Source: CAD feature listing. Evaluate the final solid. Frame: model axes, mm. Face numbers are marked on the shaded views. A direction names the side the tool comes from. Coordinates: 2 decimals unless noted, no trailing zeros. Order: outer loops, then holes, each group sorted by start corner. A loop starts at its lowest first (then second) coordinate and runs counter-clockwise, first axis right, second up.
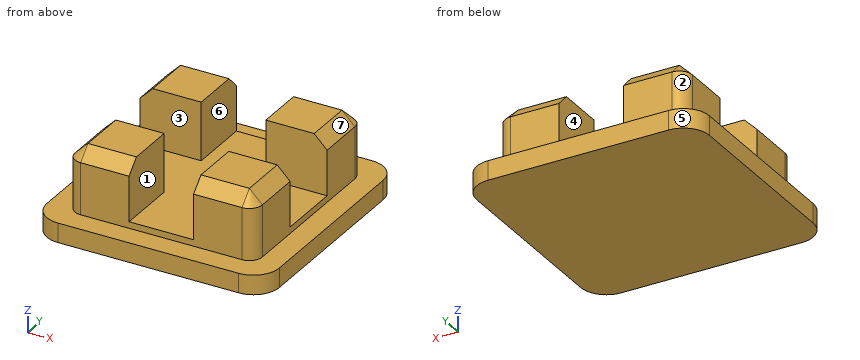
```python
from build123d import *

# Parameters (mm, degrees)
F1_DEPTH = 3
F3_DEPTH = 10
F5_DEPTH = 9
F6_SIZE  = 1.99999


# Not quite as in the source:
# - a fillet or chamfer is up to 0.001 mm smaller than in the source, because OpenCascade refuses the exact size


with BuildPart() as f1:
    # F0 (on Top) → F1 (new body)
    with BuildSketch(Plane.XY):
        with BuildLine():
            Line((16.3916659281, 18.4843443355), (-11.6083340719, 18.4843443355))
            ThreePointArc((-11.6083340719, 18.4843443355), (-14.4367611967, 17.3127714603), (-15.6083340719, 14.4843443355))
            Line((-15.6083340719, 14.4843443355), (-15.6083340719, -13.5156556645))
            ThreePointArc((-15.6083340719, -13.5156556645), (-14.4367611967, -16.3440827892), (-11.6083340719, -17.5156556645))
            Line((-11.6083340719, -17.5156556645), (16.3916659281, -17.5156556645))
            ThreePointArc((16.3916659281, -17.5156556645), (19.2200930528, -16.3440827892), (20.3916659281, -13.5156556645))
            Line((20.3916659281, -13.5156556645), (20.3916659281, 14.4843443355))
            ThreePointArc((20.3916659281, 14.4843443355), (19.2200930528, 17.3127714603), (16.3916659281, 18.4843443355))
        make_face()
    extrude(amount=F1_DEPTH)

    # F2 (on face) → F3 (join)
    with BuildSketch(Plane.XY.offset(3)):
        with BuildLine():
            Line((14.8916659281, 14.9843443355), (-10.1083340719, 14.9843443355))
            ThreePointArc((-10.1083340719, 14.9843443355), (-11.5225476343, 14.3985578979), (-12.1083340719, 12.9843443355))
            Line((-12.1083340719, 12.9843443355), (-12.1083340719, -12.0156556645))
            ThreePointArc((-12.1083340719, -12.0156556645), (-11.5225476343, -13.4298692268), (-10.1083340719, -14.0156556645))
            Line((-10.1083340719, -14.0156556645), (14.8916659281, -14.0156556645))
            ThreePointArc((14.8916659281, -14.0156556645), (16.3058794904, -13.4298692268), (16.8916659281, -12.0156556645))
            Line((16.8916659281, -12.0156556645), (16.8916659281, 12.9843443355))
            ThreePointArc((16.8916659281, 12.9843443355), (16.3058794904, 14.3985578979), (14.8916659281, 14.9843443355))
        make_face()
    extrude(amount=F3_DEPTH)

    # F4 (on face) → F5 (cut)
    with BuildSketch(Plane.XY.offset(13)):
        Polygon((7.3916660622, 14.9843443355), (-2.6083340719, 14.9843443355), (-2.6083340719, 5.4843444377), (-12.1083340719, 5.4843444377), (-12.1083340719, -4.5156556645), (-2.6083340719, -4.5156556645), (-2.6083340719, -14.0156556645), (7.3916660622, -14.0156556645), (7.3916660622, -4.5156556645), (16.8916659281, -4.5156556645), (16.8916659281, 5.4843444377), (7.3916660622, 5.4843444377), align=None)
    extrude(amount=-F5_DEPTH, mode=Mode.SUBTRACT)

    # F6 (size 2 in the source; OpenCascade refuses exactly that, so slightly less here)
    f6_edges = [f1.edges().sort_by_distance(p)[0] for p in [
        (11.141666, -14.015656, 13),
        (-6.358334, -14.015656, 13),
        (16.891666, 9.234344, 13),
        (-12.108334, 9.234344, 13),
    ]]
    chamfer(f6_edges, length=F6_SIZE)


solid = f1.part
```
1. Section query C-C, the plane y = -8.5. Output: boundary loops of the cut face in (x, z).
2. Contact query for flat-ended pins moving along their axis: P1, Ø6.5, axis at x = 8, z = 8, coming from the +Y side; P2, Ø4.5, axis at y = -11.5, z = 9, coming from the +X side; P3, Ø2.5, axis at y = -9, z = 10.5, coming from the -X side. Output: stop coordinate, or through.
3. Section query B-B, the plane x = 8. Output: boundary loops of the cut face in (y, z), plus the area to 3 significant figures.
4. Section query A-A, the plane z = 5.25. Output: boundary loops of the cut face in (x, y), plus the area to 3 significant figures.
5. Material intervals for line 1 along Y through (x, z) = (-6.5, 10.5); line 2 along X through (y, z) = (8, 4.5); line 3 along X through (y, z) = (-7, 11.5), sorted ascending.
6. Access query for the marked faces 1, 2 and 3. Directions: +Z, -Z, +X, -X, +Y, -Y. A direction counts if a zero-diameter tool reaches every point of the face in a straight line with its end or side. Return the directions, or none.
7. Section query D-D, the plane x = 2. Output: boundary loops of the cut face in (y, z), plus the area to 3 significant figures.
8. Draft query along X for the marked faces 4, 5, 6 and 7. Return one class per face: +X half, -X half, draft (parallel to the pull), parting line (faces both ways), or undercut.
Answer key:
1. outline: (-15.61, 0) - (20.39, 0) - (20.39, 3) - (16.89, 3) - (16.89, 11) - (14.89, 13) - (7.39, 13) - (7.39, 4) - (-2.61, 4) - (-2.61, 13) - (-10.11, 13) - (-12.11, 11) - (-12.11, 3) - (-15.61, 3) - close
2. P1: stops at y = 14.98
2. P2: stops at x = 16.89
2. P3: stops at x = -12.11
3. outline: (-17.52, 0) - (18.48, 0) - (18.48, 3) - (14.98, 3) - (14.98, 11) - (12.98, 13) - (5.48, 13) - (5.48, 4) - (-4.52, 4) - (-4.52, 13) - (-12.02, 13) - (-14.02, 11) - (-14.02, 3) - (-17.52, 3) - close
3. area: 304 mm2
4. outline: (-12.11, -12.02) arc R2 ccw to (-10.11, -14.02) - (-2.61, -14.02) - (-2.61, -4.52) - (-12.11, -4.52) - close; (-12.11, 5.48) - (-2.61, 5.48) - (-2.61, 14.98) - (-10.11, 14.98) arc R2 ccw to (-12.11, 12.98) - close; (7.39, -14.02) - (14.89, -14.02) arc R2 ccw to (16.89, -12.02) - (16.89, -4.52) - (7.39, -4.52) - close; (7.39, 5.48) - (16.89, 5.48) - (16.89, 12.98) arc R2 ccw to (14.89, 14.98) - (7.39, 14.98) - close
4. area: 358 mm2
5. line 1: y = -14.02 to -4.52, 5.48 to 14.98
5. line 2: x = -12.11 to -2.61, 7.39 to 16.89
5. line 3: x = -11.61 to -2.61, 7.39 to 16.39
6. face 1: +Z, +Y, -Y
6. face 2: +Z, -X, +Y
6. face 3: +Z, +X, -X
7. outline: (-17.52, 0) - (18.48, 0) - (18.48, 3) - (14.98, 3) - (14.98, 4) - (-14.02, 4) - (-14.02, 3) - (-17.52, 3) - close
7. area: 137 mm2
8. face 4: undercut
8. face 5: -X half
8. face 6: undercut
8. face 7: +X half
